The model under review builds one solid part; all positions refer to its coordinate system, in mm. A direction names the side the tool comes from. Give positions to 0.01 mm unless a question says otherwise; leave off trailing zeros. Order: outer loops, then holes, each group sorted by start corner. A loop starts at its lowest first (then second) coordinate and runs counter-clockwise, first axis right, second up.
```python
from build123d import *

# Parameters (mm, degrees)
CROQUIS1_R                   = 30.165
CROQUIS1_R_2                 = 5.5
CROQUIS1_R_3                 = 1.6
SALIENTE_EXTRUIR1_DEPTH      = 4.5
SALIENTE_EXTRUIR1_DEPTH_BACK = 4.5
SKETCH1_R                    = 9.5
CUT_EXTRUDE1_DEPTH           = 2.5
SKETCH2_R                    = 11
CUT_EXTRUDE2_DEPTH           = 5
CROQUIS3_R                   = 1.75


with BuildPart() as part:
    # Croquis1 → Saliente-Extruir1 (new, two sides)
    with BuildSketch(Plane.XY) as saliente_extruir1_sk:
        Circle(CROQUIS1_R)
        Circle(CROQUIS1_R_2, mode=Mode.SUBTRACT)
        with Locations((20, 0)):
            Circle(CROQUIS1_R_3, mode=Mode.SUBTRACT)
        with Locations((-20, 0)):
            Circle(CROQUIS1_R_3, mode=Mode.SUBTRACT)
        with Locations((0, 20)):
            Circle(CROQUIS1_R_3, mode=Mode.SUBTRACT)
        with Locations((0, -20)):
            Circle(CROQUIS1_R_3, mode=Mode.SUBTRACT)
    extrude(amount=SALIENTE_EXTRUIR1_DEPTH)
    extrude(saliente_extruir1_sk.sketch, amount=-SALIENTE_EXTRUIR1_DEPTH_BACK)

    # Sketch1 → Cut-Extrude1 (cut)
    with BuildSketch(Plane(origin=(0, 0, -4.5), x_dir=(-1, 0, 0), z_dir=(0, 0, -1))):
        Circle(SKETCH1_R)
    extrude(amount=-CUT_EXTRUDE1_DEPTH, mode=Mode.SUBTRACT)

    # Sketch2 → Cut-Extrude2 (cut)
    with BuildSketch(Plane.XY.offset(4.5)):
        Circle(SKETCH2_R)
    extrude(amount=-CUT_EXTRUDE2_DEPTH, mode=Mode.SUBTRACT)

    # Cortar-Barrer1: sweep along a curve in space
    with BuildLine() as cortar_barrer1_path:
        ThreePointArc((11, 0, 4.5), (7.778174593, 7.778174593, 4.5), (0, 11, 4.5))
        ThreePointArc((0, 11, 4.5), (-7.778174593, 7.778174593, 4.5), (-11, 0, 4.5))
        ThreePointArc((-11, 0, 4.5), (-7.778174593, -7.778174593, 4.5), (0, -11, 4.5))
        ThreePointArc((0, -11, 4.5), (7.778174593, -7.778174593, 4.5), (11, 0, 4.5))
    # Croquis3 → Cortar-Barrer1 (sweep, cut)
    with BuildSketch(Plane(origin=(0, 0, 0), x_dir=(0, 0, -1), z_dir=(1, 0, 0))):
        with Locations((-4.5, 15.75)):
            Circle(CROQUIS3_R)
    sweep(path=cortar_barrer1_path.line, mode=Mode.SUBTRACT)


solid = part.part
```
Item 1: For line 1 (Y direction, x = -1, z = 0.5); line 2 (Z direction, x = -7, y = -6.5); line 3 (X direction, y = 19.5, z = -1.5), list the stretches that pass through material, from the lowest coordinate up.
Values found:
line 1: y = -30.15 to -21.25, -18.75 to -10.95, 10.95 to 18.75, 21.25 to 30.15
line 2: z = -4.5 to -0.5
line 3: x = -23.01 to -1.52, 1.52 to 23.01
Item 2: Take a section at D-D (x = 26.5). Give the boundary of the cut face in (y, z), and give its area (3 significant figures).
Values found:
outline: (-14.41, -4.5) - (14.41, -4.5) - (14.41, 4.5) - (-14.41, 4.5) - close
area: 259 mm2
Item 3: Take a section at A-A (z = 2). Give the boundary of the cut face in (x, y) (3 decimals).
Values found:
outline: circle Ø60.33 at (0, 0); hole circle Ø3.2 at (-20, 0); hole circle Ø22 at (0, 0); hole circle Ø3.2 at (0, -20); hole circle Ø3.2 at (0, 20); hole circle Ø3.2 at (20, 0)
Item 4: Draft analysis for pull direction X (two halves, no side actions). For faces 1 (the cylindrical face through (-1.19, -5.37, -1.24)), 2 (the flat face through (-7, 7, -4.5)), 3 (the cylindrical face through (-23.94, -18.35, 0.06)), state which applies: released by +X, released by -X, zero draft, split by the parting line, or undercut.
Values found:
face 1: undercut
face 2: zero draft
face 3: split by the parting line
Item 5: For faces 4 (the flat face through (6.2, -9.3, 4.5)), 5 (the cylindrical face through (-2.38, -10.74, 2.04)), 6 (the flat face through (-4, -4, -2)), list the 3-axis set-ups (+Z, -Z, +X, -X, +Y, -Y) from which the entire face can be reached by the end or side of a thin tool; tool diameter is ignored.
Values found:
face 4: +Z, +X, -X, +Y, -Y
face 5: +Z
face 6: -Z
Item 6: Take a section at B-B (x = 20). Give the boundary of the cut face in (y, z).
Values found:
outline: (-22.58, -4.5) - (-1.6, -4.5) - (-1.6, 4.5) - (-22.58, 4.5) - close; (1.6, -4.5) - (22.58, -4.5) - (22.58, 4.5) - (1.6, 4.5) - close
Item 7: Clearance check with flat-ended pins moving along their axes: pin 1 Ø1 at (y, z) = (-15, 0.5) entering from -X; pin 2 Ø11.5 at (x, y) = (0, 0) entering from +Z; pin 3 Ø4 at (y, z) = (13.5, 2) entering from -X; pin 4 Ø2.5 at (x, y) = (-20, 0) entering from +Z. State where each tip first meets the part, or that it passes through.
Values found:
pin 1: stops at x = -26.45
pin 2: stops at z = -0.5
pin 3: stops at x = -27.89
pin 4: passes through
